Could you check a few things on this model? Use its own coordinates, in mm. A direction names the side the tool comes from. Give positions to 0.01 mm unless a question says otherwise; leave off trailing zeros. Loops run counter-clockwise (first coordinate to the right, second up) from the corner with the lowest first, then second, coordinate; pieces in that order, holes last. Notation, with made-up numbers: M 64,-14 L 90,-14 A11 ccw 90,3 Z; hole C -26.5,-20.5 d11. An arc over 180 degrees is marked long. Answer in a Markdown table with one row per item. Add a question column.
Solid Edge part; units mm, degrees
sketch "Sketch1" plane through (0, 0, 0) normal (0, 0, 1) x (1, 0, 0)
  line L0 (-30, -13.905) -> (30, -13.905)
  line L1 (30, -13.905) -> (30, 13.905)
  line L2 (30, 13.905) -> (-30, 13.905)
  line L3 (-30, 13.905) -> (-30, -13.905)
  dimension "D1" = 30
  dimension "D2" = 30
extrude "Protrusion1" add sketch "Sketch1" along normal blind 2
sketch "Sketch2" plane through (0, 0, 2) normal (0, 0, 1) x (1, 0, 0)
  line L0 (30, 13.905) -> (-12.5, 13.905)
  line L1 (-12.5, 13.905) -> (-12.5, 23.095)
  line L2 (-12.5, 23.095) -> (30, 23.095)
  line L3 (30, 23.095) -> (30, 13.905)
  dimension "D1" = 30
  dimension "D2" = 12.5
extrude "Extrusionsausprägung_2" add sketch "Sketch2" against normal blind 2
sketch "Sketch3" plane through (0, 4.595, 2) normal (0, 0, 1) x (1, 0, 0)
  circle A0 centre (-25, -5.5) radius 1.1
  circle A1 centre (27.5, 10.5) radius 1.1
  circle A2 centre (27.5, -2.5) radius 1.1
  dimension "D1" = 25
extrude "Cutout1" cut sketch "Sketch3" against normal up to next
sketch "Sketch4" plane through (-30, 0, 1) normal (-1, 0, 0) x (0, -1, 0)
  line L0 (-13.905, 1) -> (-13.905, 9.1)
  line L1 (-13.905, 9.1) -> (-11.905, 9.1)
  arc A0 (-11.905, 9.1) -> (-6.905, 5.05) centre (-11.905, 3.98858) cw
  arc A1 (-6.905, 5.05) -> (-1.905, 1) centre (-1.905, 6.11142) ccw
  line L2 (-13.905, 1) -> (-1.905, 1)
  dimension "D1" = 13.905
  dimension "D2" = 13.905
  dimension "D3" = 13.905
extrude "Extrusionsausprägung_3" add sketch "Sketch4" against normal blind 17.5
fillet "Verrundung_1" radius 2 1 edges at (0, -13.905, 2)
mirror "Mirror1" about plane through (0, 0, 0) normal (1, 0, 0) of "Extrusionsausprägung_3"
sketch "Sketch5" plane through (21.25, 12.905, 10.1) normal (0, 0, 1) x (-1, 0, 0)
  circle A0 centre (-6.25, -2.19) radius 5
extrude "Cutout2" cut sketch "Sketch5" against normal up to vertex (8.1 mm away)
sketch "Sketch6" plane through (-24, 10.405, 2) normal (0, 0, 1) x (-1, 0, 0)
  circle A0 centre (0, -0.69) radius 1.1
extrude "Cutout3" cut sketch "Sketch6" against normal through all
sketch "Sketch7" plane through (-21.25, 12.905, 10.1) normal (0, 0, 1) x (-1, 0, 0)
  circle A0 centre (2.75, 1.81) radius 5
extrude "Cutout4" cut sketch "Sketch7" against normal up to vertex (8.1 mm away)
Item 1: For faces 1 (the face through (-12.5, 10, 5)), 2 (the face through (-12.5, 18, 1)), 3 (the face through (26.627, 1.426, 1.014)), which set-ups out of +Z, -Z, +X, -X, +Y, -Y let a thin tool reach every point of the face, with its end or its side?
Item 2: I need wall thicknesses on L1, parallel to X at y = 10, z = 3.25; L2, parallel to Y at x = 27.5, z = 1.1 (3 decimals); L3, parallel to Z at x = 20.5, y = -6.5. Which ranges of each line are inside material? Lowest first, please.
Item 3: Suppose I cut it at C-C (z = 1.25). List the corners of the cut face in (x, y) for me (3 decimals), then the cut area to 3 significant figures.
Item 4: If we mould it in two halves opening along Y, with no side actions, what happens to faces 4 (the face through (12.5, 10, 5)), 5 (the face through (-26.45, 6.736, 4.307)), 6 (the face through (25.48, 10.52, 6.11))? For each: +Y half, -Y half, draft (parallel to the pull), parting line (faces both ways), or undercut.
Item 5: Suppose I cut it at A-A (z = 8.25). List the corners of the cut face in (x, y) for me (3 decimals), then the cut area to 3 significant figures.
Item 6: Suppose I cut it at D-D (y = 4). List the corners of the cut face in (x, z) for me.
Item 7: For P1, Ø1.5, axis at x = -0.5, z = 1, coming from the -Y side; P2, Ø0.6, axis at x = 28, y = 2.5, coming from the -Z side; P3, Ø2, axis at x = 27.5, y = 2.095, coming from the +Z side, each with a flat end and sliding along its axis, tell me the tip position at first contact or that it passes through.
Values found:
| question | item | result |
|---|---|---|
| 1 | face 1 | +Z, +Y, -Y |
| 1 | face 2 | +Z, -Z, -X, +Y |
| 1 | face 3 | -Z |
| 2 | L1 | -30 to -28.88, -19.12 to -12.5, 12.5 to 30 |
| 2 | L2 | -13.575 to 0.995, 3.195 to 13.995, 16.195 to 23.095 |
| 2 | L3 | 0 to 2 |
| 3 | outline | M -30,-13.466 L 30,-13.466 L 30,23.095 L -12.5,23.095 L -12.5,13.905 L -30,13.905 Z; hole C -25,-0.905 d2.2; hole C -24,11.095 d2.2; hole C 27.5,2.095 d2.2; hole C 27.5,15.095 d2.2 |
| 3 | area | 2,020 mm² |
| 4 | face 4 | draft |
| 4 | face 5 | undercut |
| 4 | face 6 | +Y half |
| 5 | outline | M -30,7.969 L -27.903,7.969 A5 cw -28.136,13.905 L -30,13.905 Z; M -20.097,7.969 L -12.5,7.969 L -12.5,13.905 L -19.864,13.905 A5 cw Z; M 12.5,7.969 L 30,7.969 L 30,10.765 A5 cw 22.644,13.905 L 12.5,13.905 Z |
| 5 | area | 129 mm² |
| 6 | outline | M -30,0 L 30,0 L 30,2.45 L 12.5,2.45 L 12.5,2 L -12.5,2 L -12.5,2.45 L -30,2.45 Z |
| 7 | P1 | y = -13.89 |
| 7 | P2 | z = 2 |
| 7 | P3 | z = 2.14 |
